Autodesk Inventor part; units mm, degrees
ref_plane "YZ Plane" through (0, 0, 0) normal (1, 0, 0) x (0, 1, 0)
ref_plane "XZ Plane" through (0, 0, 0) normal (0, 1, 0) x (-1, 0, 0)
ref_plane "XY Plane" through (0, 0, 0) normal (0, 0, 1) x (1, 0, 0)
sketch "Эскиз1" plane through (0, 0, 0) normal (1, 0, 0) x (0, 1, 0)
  line L0 (-30, 0) -> (30, 0)
  line L1 (-30, 0) -> (-30, 40)
  line L2 (-30, 40) -> (-12, 40)
  line L3 (30, 0) -> (30, 27.5)
  line L4 (30, 27.5) -> (0, 27.5)
  line L5 (0, 27.5) -> (-12, 40)
  circle A0 centre (-18, 28) radius 4
  line L6 (-30, 0) -> (-30, -40)
  line L7 (-30, -40) -> (-12, -40)
  line L8 (30, 0) -> (30, -27.5)
  line L9 (30, -27.5) -> (0, -27.5)
  line L10 (0, -27.5) -> (-12, -40)
  circle A1 centre (-18, -28) radius 4
  point P0 (0, 0)
  point P1 (0, 0)
  dimension "d1" = 40
  dimension "d2" = 18
  dimension "d3" = 55
  dimension "d4" = 30
  dimension "d5" = 60
  dimension "d6" = 8
  dimension "d7" = 12
  dimension "d8" = 12
extrude "Выдавливание1" add sketch "Эскиз1" along normal blind 2
properties part number "Для иконки" material "Медь"
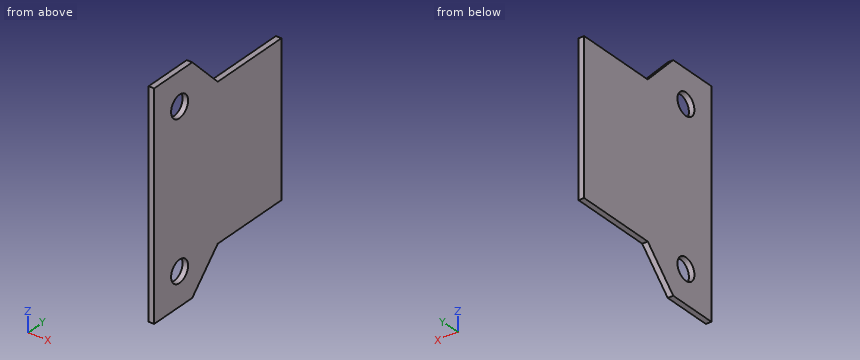
Geometry check sheet. Reference: the model listing, model coordinates, mm. Coordinates: 2 decimals unless noted, no trailing zeros. Order: outer loops, then holes, each group sorted by start corner. A loop starts at its lowest first (then second) coordinate and runs counter-clockwise, first axis right, second up. Notation, with made-up numbers: (69.5, 44.25) - (77.5, 44.25) arc R16 ccw to (77.5, 63.25) - close; hole circle Ø7 at (56.5, 65.5). An arc over 180 degrees is marked (long way). Answer in a Markdown table with one row per item. Add a question column.
1. Section check A-A (y = -18). Enter the section's corners in (x, z).
2. Material ranges on L1, parallel to Z at x = 1.2, y = -18; L2, parallel to Z at x = 1.65, y = 22; L3, parallel to Y at x = 0.8, z = -26.5, recorded low to high. Write a range as [from, to].
3. Section check C-C (z = -34). Enter the section's corners in (x, y), plus the area to 3 significant figures.
4. Section check D-D (y = 7.5). Enter the section's corners in (x, z).
5. Gauge pin test, flat ends, axial feed: pin 1 Ø0.6 at (x, y) = (1, 17) entering from -Z; pin 2 Ø5 at (y, z) = (-18, -28) entering from +X. Record the tip position at first contact, or that the pin passes through.
6. Section check B-B (x = 1.6). Enter the section's corners in (y, z).
Data:
| question | item | result |
|---|---|---|
| 1 | outline | (0, -40) - (2, -40) - (2, -32) - (0, -32) - close; (0, -24) - (2, -24) - (2, 24) - (0, 24) - close; (0, 32) - (2, 32) - (2, 40) - (0, 40) - close |
| 2 | L1 | z = [-40, -32], [-24, 24], [32, 40] |
| 2 | L2 | z = [-27.5, 27.5] |
| 2 | L3 | y = [-30, -21.71], [-14.29, 30] |
| 3 | outline | (0, -30) - (2, -30) - (2, -6.24) - (0, -6.24) - close |
| 3 | area | 47.5 mm² |
| 4 | outline | (0, -27.5) - (2, -27.5) - (2, 27.5) - (0, 27.5) - close |
| 5 | pin 1 | stops at z = -27.5 |
| 5 | pin 2 | passes through |
| 6 | outline | (-30, -40) - (-12, -40) - (0, -27.5) - (30, -27.5) - (30, 27.5) - (0, 27.5) - (-12, 40) - (-30, 40) - close; hole circle Ø8 at (-18, -28); hole circle Ø8 at (-18, 28) |
